Here's how the part is built. I have some questions about the finished solid (model axes, mm). Round coordinates to 2 decimals unless told otherwise and drop trailing zeros. Loops run counter-clockwise (first coordinate to the right, second up) from the corner with the lowest first, then second, coordinate; pieces in that order, holes last. Notation, with made-up numbers: M 27,33 L 69,33 A34 cw 69,69 Z; hole C 76.25,83.5 d3. An arc over 180 degrees is marked long. Use a Markdown table: item, result.
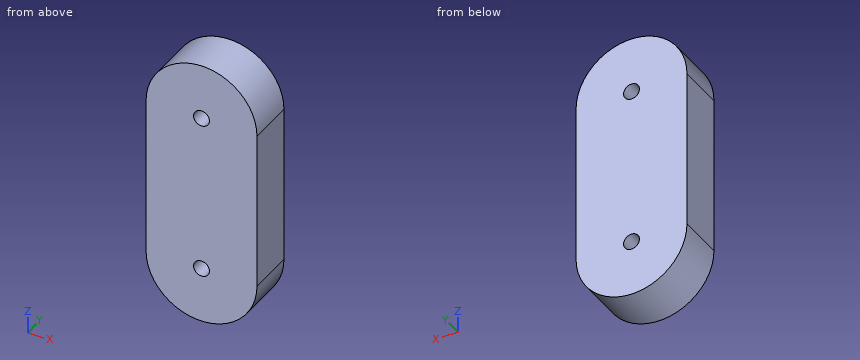
from build123d import *

# Parameters (mm, degrees)
F1_DEPTH = 38.1
F2_D     = 12.7


# Not quite as in the source:
# - a length typed as a fraction of an inch, garbled in the dataset ("3 / 203.2 mm" for 3/8 in), is restored


with BuildPart() as f1:
    # F0 (on Front) → F1 (new body)
    with BuildSketch(Plane.XZ):
        with BuildLine():
            Line((44.45, -63.5), (44.45, 63.5))
            ThreePointArc((44.45, 63.5), (0, 107.95), (-44.45, 63.5))
            Line((-44.45, 63.5), (-44.45, -63.5))
            ThreePointArc((-44.45, -63.5), (0, -107.95), (44.45, -63.5))
        make_face()
    extrude(amount=F1_DEPTH)

    # F2 (through all)
    with Locations(Plane(origin=(0, 0, 0), x_dir=(1, 0, 0), z_dir=(0, 1, 0))):
        with Locations((0, -63.5), (0, 63.5)):
            Hole(F2_D / 2)


solid = f1.part
1. Imagine slicing it at D-D, the plane x = -34. Write out the boundary of the cut face in (y, z).
Answer sheet:
| item | result |
|---|---|
| outline | M -38.1,-92.13 L 0,-92.13 L 0,92.13 L -38.1,92.13 Z |
2. I need wall thicknesses on probe 1 along Z at (x, y) = (0, -16.5); probe 2 along X at (y, z) = (-14, -63.5); probe 3 along Z at (x, y) = (-34, -11.5). Which ranges of each line are inside material? Lowest first, please. Write a range as from..to.
Answer sheet:
| item | result |
|---|---|
| probe 1 | -107.95..-69.85, -57.15..57.15, 69.85..107.95 |
| probe 2 | -44.45..-6.35, 6.35..44.45 |
| probe 3 | -92.13..92.13 |
3. For pin 1 Ø3 at (x, y) = (-16.5, -31) entering from -Z; pin 2 Ø5 at (y, z) = (-34, -80) entering from -X, each with a flat end and sliding along its axis, tell me the tip position at first contact or that it passes through.
Answer sheet:
| item | result |
|---|---|
| pin 1 | z = -105.34 |
| pin 2 | x = -42.19 |
4. Imagine slicing it at A-A, the plane x = 0. Write out the boundary of the cut face in (y, z).
Answer sheet:
| item | result |
|---|---|
| outline | M -38.1,-107.95 L 0,-107.95 L 0,-69.85 L -38.1,-69.85 Z; M -38.1,-57.15 L 0,-57.15 L 0,57.15 L -38.1,57.15 Z; M -38.1,69.85 L 0,69.85 L 0,107.95 L -38.1,107.95 Z |
5. Imagine slicing it at B-B, the plane y = -5. Write out the boundary of the cut face in (x, z).
Answer sheet:
| item | result |
|---|---|
| outline | M -44.45,-63.5 A44.45 ccw 44.45,-63.5 L 44.45,63.5 A44.45 ccw -44.45,63.5 Z; hole C 0,-63.5 d12.7; hole C 0,63.5 d12.7 |
6. Imagine slicing it at C-C, the plane z = 67. Write out the boundary of the cut face in (x, y).
Answer sheet:
| item | result |
|---|---|
| outline | M -44.31,-38.1 L -5.3,-38.1 L -5.3,0 L -44.31,0 Z; M 5.3,-38.1 L 44.31,-38.1 L 44.31,0 L 5.3,0 Z |
